The model under review builds one solid part; all positions refer to its coordinate system, in mm. A direction names the side the tool comes from. Round coordinates to 2 decimals unless told otherwise and drop trailing zeros. Write each loop counter-clockwise with the first axis right and the second up, starting at its lowest first coordinate (ties: lowest second). Pieces come first, ordered by that corner, then holes. Notation, with made-up numbers: (-36.75, 13.25) - (-17.75, 13.25) arc R25 ccw to (-17.75, 46.25) - close; hole circle Ø5 at (15.5, 59). An arc over 180 degrees is marked (long way). One line per question, with ' | ' between items. Start each with the question number.
```python
from build123d import *

# Parameters (mm, degrees)
F1_DEPTH = 16


with BuildPart() as f1:
    # F0 (on Front) → F1 (new body)
    with BuildSketch(Plane.XZ):
        with BuildLine():
            ThreePointArc((0, -9), (-9, 0), (0, 9))
            Line((0, 9), (94, 9))
            Line((94, 9), (94, 11))
            Line((94, 11), (0, 11))
            ThreePointArc((0, 11), (-11, 0), (0, -11))
            Line((0, -11), (19, -11))
            ThreePointArc((19, -11), (20.746435, -11.560745), (21.84, -13.033356))
            ThreePointArc((21.84, -13.033356), (38.975661, -40.632695), (66.498813, -57.89046))
            ThreePointArc((66.498813, -57.89046), (70.094434, -59.751434), (73.007182, -62.563483))
            Line((73.007182, -62.563483), (74.3191, -61))
            ThreePointArc((74.3191, -61), (71.083349, -58.001162), (67.151624, -56))
            ThreePointArc((67.151624, -56), (40.393003, -39.221618), (23.733333, -12.388927))
            ThreePointArc((23.733333, -12.388927), (21.910725, -9.934575), (19, -9))
            Line((19, -9), (0, -9))
        make_face()
    extrude(amount=F1_DEPTH)


solid = f1.part
```
1. Add section B-B, the plane y = -13. Write out the cut boundary in (x, z), then the cut area to 3 significant figures.
2. The part is to be moulded in two halves that separate along Z. For faces 1 (the face through (48, -8, 11)), 2 (the face through (22, -8, -10)), 3 (the face through (94, -8, 10)), 4 (the face through (38.653, -7.888, -40.307)), say which applies: pulls with the +Z half, pulls with the -Z half, needs draft (parallel to the pull), parting line crosses it, or undercut.
3. Wall thickness on line 1 along Z through (x, y) = (5.5, -2.75); line 2 along X through (y, z) = (-2.5, 0); line 3 along Z through (x, y) = (42.5, -6.5): over which ranges is each line inside the solid? List them lowest first. Write a range as [from, to].
4. Add section A-A, the plane x = 40.5. Write out the cut boundary in (y, z).
5. Add section C-C, the plane z = 0. Write out the cut boundary in (x, y), then the cut area to 3 significant figures.
6. Machinability: for faces 5 (the face through (-11, -8, 0)), 6 (the face through (9, -8, -11)), 7 (the face through (40.71, -7.89, -39.54)), which of the approach directions +Z, -Z, +X, -X, +Y, -Y give a long, thin tool a straight path to every point of the face, cutting with its end or side? Answer none if there is none.
7. Clearance check with flat-ended pins moving along their axes: P1, Ø5, axis at y = -8, z = -25.5, coming from the -X side; P2, Ø3, axis at y = -10, z = -50.5, coming from the +X side; P3, Ø5, axis at y = -3, z = -52.5, coming from the -X side; P4, Ø12, axis at x = 22.5, z = -15, coming from the -Y side. State where each tip first meets the part, or that it passes through.
8. Add section D-D, the plane x = 75.5. Write out the cut boundary in (y, z), then the cut area to 3 significant figures.
Geometry check:
1) outline: (0, -11) - (19, -11) arc R3 cw to (21.84, -13.03) arc R72 ccw to (66.5, -57.89) arc R14 cw to (73.01, -62.56) - (74.32, -61) arc R16 ccw to (67.15, -56) arc R70 cw to (23.73, -12.39) arc R5 ccw to (19, -9) - (0, -9) arc R9 cw to (0, 9) - (94, 9) - (94, 11) - (0, 11) arc R11 ccw to start | area: 445 mm2
2) face 1: pulls with the +Z half | face 2: undercut | face 3: needs draft | face 4: pulls with the -Z half
3) line 1: z = [-11, -9], [9, 11] | line 2: x = [-11, -9] | line 3: z = [-43.94, -41.25], [9, 11]
4) outline: (-16, -42.12) - (0, -42.12) - (0, -39.33) - (-16, -39.33) - close; (-16, 9) - (0, 9) - (0, 11) - (-16, 11) - close
5) outline: (-11, -16) - (-9, -16) - (-9, 0) - (-11, 0) - close | area: 32.0 mm2
6) face 5: -X, +Y, -Y | face 6: -Z, -X, +Y, -Y | face 7: +X, +Y, -Y
7) P1: stops at x = 26.09 | P2: stops at x = 57.82 | P3: stops at x = 50.45 | P4: stops at y = -16
8) outline: (-16, 9) - (0, 9) - (0, 11) - (-16, 11) - close | area: 32.0 mm2
